Autodesk Inventor part; units mm, degrees
ref_plane "YZ Plane" through (0, 0, 0) normal (1, 0, 0) x (0, 1, 0)
ref_plane "XZ Plane" through (0, 0, 0) normal (0, 1, 0) x (-1, 0, 0)
ref_plane "XY Plane" through (0, 0, 0) normal (0, 0, 1) x (1, 0, 0)
sketch "Sketch1" plane through (0, 0, 0) normal (0, 0, 1) x (1, 0, 0)
  line L0 (-26.6827, 34.4805) -> (26.6827, 34.4805)
  line L1 (26.6827, 34.4805) -> (26.6827, -34.4805)
  line L2 (26.6827, -34.4805) -> (-26.6827, -34.4805)
  line L3 (-26.6827, -34.4805) -> (-26.6827, 34.4805)
  circle A0 centre (24.0919, -18.8595) radius 1.5113
  circle A1 centre (-24.0919, -20.5105) radius 1.5113
  circle A2 centre (-8.7503, 32.0675) radius 1.5113
  circle A3 centre (18.6563, 32.0675) radius 1.5113
  point P0 (0, 0)
  dimension "d0" = 53.3654
  dimension "d1" = 68.961
  dimension "d2" = 3.0226
  dimension "d3" = 3.0226
  dimension "d4" = 15.621
  dimension "d5" = 13.97
  dimension "d6" = 2.5908
  dimension "d7" = 2.5908
  dimension "d8" = 3.0226
  dimension "d9" = 3.0226
  dimension "d11" = 17.9324
  dimension "d12" = 8.0264
  dimension "d13" = 2.413
extrude "Extrusion1" add sketch "Sketch1" along normal blind 13.4112
sketch "Sketch2" plane through (-26.6827, -34.4805, 0) normal (0, -1, 0) x (1, 0, 0)
  line L0 (0, 0) -> (53.3654, 0)
  line L1 (8.9662, 13.4061) -> (21.082, 13.4061)
  line L2 (21.082, 13.4061) -> (21.082, 2.6111)
  line L3 (21.082, 2.6111) -> (8.9662, 2.6111)
  line L4 (8.9662, 2.6111) -> (8.9662, 13.4061)
  line L5 (8.9662, 13.4061) -> (21.082, 2.6111) construction
  line L6 (21.082, 13.4061) -> (8.9662, 2.6111) construction
  line L7 (0, 0) -> (0, 13.4112)
  point P0 (26.6827, 0)
  point P1 (15.0241, 8.0086)
  dimension "d16" = 12.1158
  dimension "d17" = 10.795
  dimension "d18" = 8.9662
extrude "Extrusion2" add sketch "Sketch2" along normal blind 6.2992
properties part number "arduino uno"
CAD build for the part. Positions are in the model's coordinates, mm. A direction names the side the tool comes from. Coordinates: 2 decimals unless noted, no trailing zeros. Loops run counter-clockwise (first coordinate to the right, second up) from the corner with the lowest first, then second, coordinate; pieces in that order, holes last. Notation, with made-up numbers: (1, 63) - (60, 63) arc R34 ccw to (60, 95) - close; hole circle Ø11 at (25, 51.25). An arc over 180 degrees is marked (long way). Write item = value, one per line. Start each with the question number.
Q1. Pull direction Y, two halves, no side cores. Call faces 6 (the flat face through (0, 34.48, 7)), 7 (the cylindrical face through (23.9, -20.36, 6.61)), 8 (the flat face through (-12, -38, 13.406)), 9 (the cylindrical face through (17.46, 32.99, 6.61)): pulls with the +Y half, pulls with the -Y half, needs draft (parallel to the pull), parting line crosses it, or undercut.
Q2. Which spindle directions (+Z, -Z, +X, -X, +Y, -Y) get a long thin tool onto all of the face, cutting with end or side? Do faces 1 (the cylindrical face through (-8.053, 33.408, 6.612)), 2 (the flat face through (-5.601, -38, 8)), 3 (the flat face through (0, 0, 0)), 4 (the flat face through (-17.716, -38, 8)), 5 (the flat face through (-12, -38, 2.611)). Say none if no direction does.
Q3. Cut at A-A, the plane z = 9. List the corners of the cut face in (x, y).
Q4. Flat gauge pins, fed straight in: pin 1 Ø5 at (y, z) = (-38, 7) entering from -X; pin 2 Ø4 at (x, y) = (-24.09, -20.51) entering from -Z; pin 3 Ø3 at (x, y) = (-10.5, -37) entering from -Z; pin 4 Ø3 at (x, z) = (20, 9.5) entering from -Y. Where does each tip first touch, or does it go through?
Q5. Drill centre lines: L1, parallel to Y at x = 9, z = 9.25; L2, parallel to X at y = -37, z = 4.5; L3, parallel to Y at x = -9, z = 5.5. Where is each one in solid material? Low to high.
Q6. Cut at B-B, the plane x = 14. List the corners of the cut face in (y, z).
Computed:
q1.face_6 = pulls with the +Y half
q1.face_7 = undercut
q1.face_8 = needs draft
q1.face_9 = undercut
q2.face_1 = +Z, -Z
q2.face_2 = +Z, -Z, +X, -Y
q2.face_3 = -Z, +X, -X, +Y, -Y
q2.face_4 = +Z, -Z, -X, -Y
q2.face_5 = -Z, +X, -X, -Y
q3.outline = (-26.68, -34.48) - (-17.72, -34.48) - (-17.72, -40.78) - (-5.6, -40.78) - (-5.6, -34.48) - (26.68, -34.48) - (26.68, 34.48) - (-26.68, 34.48) - close; hole circle Ø3.02 at (-24.09, -20.51); hole circle Ø3.02 at (-8.75, 32.07); hole circle Ø3.02 at (18.66, 32.07); hole circle Ø3.02 at (24.09, -18.86)
q4.pin_1 = -17.72
q4.pin_2 = 0
q4.pin_3 = 2.61
q4.pin_4 = -34.48
q5.L1 = -34.48 to 34.48
q5.L2 = -17.72 to -5.6
q5.L3 = -40.78 to 30.58, 33.56 to 34.48
q6.outline = (-34.48, 0) - (34.48, 0) - (34.48, 13.41) - (-34.48, 13.41) - close
